from build123d import *

# Parameters (mm, degrees)
F0_W     = 66
F0_H     = 46
F1_DEPTH = 25
F2_SIZE  = 20
F3_T     = -2.5
F4_W     = 10.88829
F4_H     = 42.176487
F5_DEPTH = 4.1


with BuildPart() as f1:
    # F0 (on Top) → F1 (new body)
    with BuildSketch(Plane.XY):
        with Locations((33, 0)):
            Rectangle(F0_W, F0_H)
    extrude(amount=F1_DEPTH)

    # F2
    f2_edges = [f1.edges().sort_by_distance(p)[0] for p in [
        (0, 0, 25),
    ]]
    chamfer(f2_edges, length=F2_SIZE)

    # F3
    f3_openings = [f1.faces().sort_by_distance(p)[0] for p in [
        (66, 0, 12.5),
    ]]
    offset(amount=F3_T, openings=f3_openings)

    # F4 (on face) → F5 (cut)
    with BuildSketch(Plane(origin=(0, 0, 0), x_dir=(1, 0, 0), z_dir=(0, 0, -1))):
        with Locations((7.093375, -0.062578)):
            Rectangle(F4_W, F4_H)
    extrude(amount=-F5_DEPTH, mode=Mode.SUBTRACT)


solid = f1.part
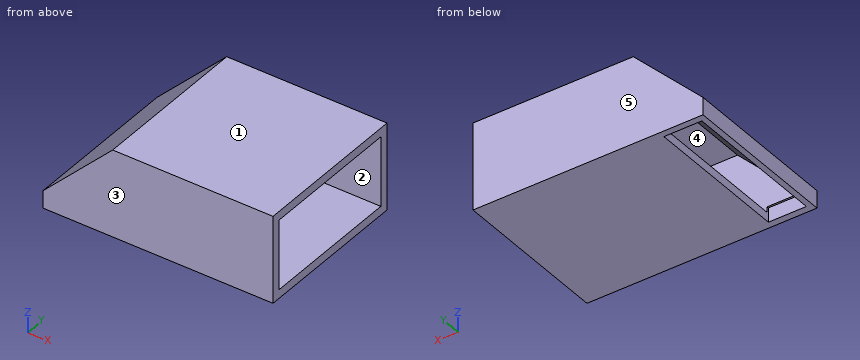
Source: CAD feature listing. Evaluate the final solid. Frame: model axes, mm. Face numbers are marked on the shaded views. A direction names the side the tool comes from. Give positions to 0.01 mm unless a question says otherwise; leave off trailing zeros. Order: outer loops, then holes, each group sorted by start corner. A loop starts at its lowest first (then second) coordinate and runs counter-clockwise, first axis right, second up. Notation, with made-up numbers: (83.25, 18.5) -> (141.25, 18.5) arc R17 cw to (141.25, 32.5) -> close; hole circle Ø4 at (-37, -25). An arc over 180 degrees is marked (long way). Write item = value, one per line.
Q1. Cut plane D-D, the plane x = 8.5. Output: boundary loops of the cut face in (y, z).
Data:
outline = (-23, 0) -> (-21.03, 0) -> (-21.03, 4.1) -> (-20.5, 4.1) -> (-20.5, 9.96) -> (20.5, 9.96) -> (20.5, 4.1) -> (21.15, 4.1) -> (21.15, 0) -> (23, 0) -> (23, 13.5) -> (-23, 13.5) -> close
Q2. Set-up query: the marked faces 1 and 2. Return all of +Z, -Z, +X, -X, +Y, -Y with unobstructed straight access to the full face (end or side cutting, diameter ignored); none if empty.
Data:
face_1 = +Z, +X, -X, +Y, -Y
face_2 = +X
Q3. Cut plane B-B, the plane x = 47.5. Output: boundary loops of the cut face in (y, z), and give its area (3 significant figures).
Data:
outline = (-23, 0) -> (23, 0) -> (23, 25) -> (-23, 25) -> close; hole (-20.5, 2.5) -> (20.5, 2.5) -> (20.5, 22.5) -> (-20.5, 22.5) -> close
area = 330 mm^2
Q4. Cut plane C-C, the plane z = 10.25. Output: boundary loops of the cut face in (x, y).
Data:
outline = (5.25, -23) -> (66, -23) -> (66, -20.5) -> (8.79, -20.5) -> (8.79, 20.5) -> (66, 20.5) -> (66, 23) -> (5.25, 23) -> close
Q5. Material intervals for line 1 (Z direction, x = 31.5, y = -14); line 2 (Y direction, x = 62, z = 20.75); line 3 (Y direction, x = 8.5, z = 3), sorted ascending. Write a range as from..to.
Data:
line_1 = 0..2.5, 22.5..25
line_2 = -23..-20.5, 20.5..23
line_3 = -23..-21.03, 21.15..23
Q6. Pull-direction query (Y, two-part tool) for the marked faces 3, 4 and 5; classes: released by +Y, released by -Y, zero draft, split by the parting line, or undercut.
Data:
face_3 = released by -Y
face_4 = undercut
face_5 = released by +Y
Q7. Pin query (flat end, axial travel): pin 1 (12 mm diameter, centred on x = 8, y = 7, fed in from -Z); pin 2 (8 mm diameter, centred on y = 9, z = 16, fed in from +X); pin 3 (1 mm diameter, centred on y = 9.5, z = 9.5, fed in from -X); pin 4 (5 mm diameter, centred on y = -5.5, z = 7, fed in from +X). Return the tip coordinate at first contact, or that it passes through.
Data:
pin_1 = 0
pin_2 = 18.54
pin_3 = 4
pin_4 = 8.04
Q8. Cut plane A-A, the plane y = 19. Output: boundary loops of the cut face in (x, z).
Data:
outline = (0, 0) -> (1.65, 0) -> (1.65, 4.1) -> (2.64, 4.1) -> (21.04, 22.5) -> (66, 22.5) -> (66, 25) -> (20, 25) -> (0, 5) -> close; (12.54, 0) -> (66, 0) -> (66, 2.5) -> (12.54, 2.5) -> close
